Geometry: final body of the model. Coordinates: model frame, mm. Face numbers are marked on the shaded views. A direction names the side the tool comes from. Round coordinates to 2 decimals unless told otherwise and drop trailing zeros. Write each loop counter-clockwise with the first axis right and the second up, starting at its lowest first coordinate (ties: lowest second). Pieces come first, ordered by that corner, then holes. Notation, with made-up numbers: M 40,-18 L 92,-18 A16 cw 92,0 Z; hole C 68.25,-13 d11. An arc over 180 degrees is marked long. Answer as CSV lines item,"result". Start each with the question number.
Q1. Ray query, probe 1 along Z at (x, y) = (2.35, -0.3); probe 2 along Z at (x, y) = (-1.85, 1.6); probe 3 along X at (y, z) = (-0.9, 1.75). Return the intervals inside material, ascending.
Q2. Reachability of the marked faces 4, 5 and 6 from +Z, -Z, +X, -X, +Y, -Y: full face, straight path, thin tool, end or side. Return the list, or none.
Q3. Section query C-C on z = 3.5. Output: boundary loops of the cut face in (x, y).
Q4. Section query B-B on x = 1.15. Output: boundary loops of the cut face in (y, z).
Q5. Section query D-D on z = 0. Output: boundary loops of the cut face in (x, y).
Q6. First-contact query: pin 1 (2.5 mm diameter, centred on x = 0, y = 0, fed in from -Z); pin 2 (2 mm diameter, centred on y = 0.5, z = -2.5, fed in from -X); pin 3 (2 mm diameter, centred on y = -1.5, z = 2.5, fed in from +X). Flat tips, straight axial feed; report the tip coordinate or a pass-through.
Q7. Mould query, pull axis Z, two halves, no side actions, for the marked faces 1, 2 and 3. Classes: pulls with the +Z half, pulls with the -Z half, needs draft (parallel to the pull), parting line crosses it, or undercut.
Q8. Section query A-A on y = 0. Output: boundary loops of the cut face in (x, z), and give its area (3 significant figures).
```python
from build123d import *


with BuildPart() as part:
    # Sketch1 → Revolve1 (revolve)
    with BuildSketch(Plane(origin=(0, 0, 0), x_dir=(1, 0, 0), z_dir=(0, 1, 0))):
        with BuildLine():
            Line((1.4732, 4.0005), (1.4732, -4.0005))
            Line((1.4732, -4.0005), (2.4892, -4.0005))
            Line((2.4892, -4.0005), (2.4892, -3.1115))
            Line((2.4892, -3.1115), (1.9304, -3.1115))
            Line((1.9304, -3.1115), (1.9304, -2.0955))
            ThreePointArc((1.9304, -2.0955), (2.849133975, 0), (1.9304, 2.0955))
            Line((1.9304, 2.0955), (1.9304, 3.1115))
            Line((1.9304, 3.1115), (2.4892, 3.1115))
            Line((2.4892, 3.1115), (2.4892, 4.0005))
            Line((2.4892, 4.0005), (1.4732, 4.0005))
        make_face()
    revolve(axis=Axis((0, 0, -2.773013621), (0, 0, 1)))


solid = part.part
```
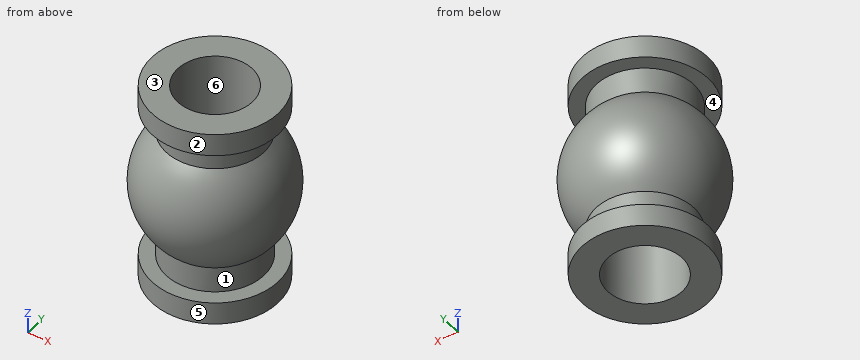
Entries:
1,probe 1,"z = -4 to -3.11, -1.58 to 1.58, 3.11 to 4"
1,probe 2,"z = -4 to -3.11, -1.46 to 1.46, 3.11 to 4"
1,probe 3,"x = -2.06 to -1.17, 1.17 to 2.06"
2,face 4,"none"
2,face 5,"-Z"
2,face 6,"+Z, -Z"
3,outline,"C 0,0 d4.98; hole C 0,0 d2.95"
4,outline,"M -2.21,-4 L -0.92,-4 L -0.92,4 L -2.21,4 L -2.21,3.11 L -1.55,3.11 L -1.55,2.1 A2.61 ccw -1.55,-2.1 L -1.55,-3.11 L -2.21,-3.11 Z; M 0.92,-4 L 2.21,-4 L 2.21,-3.11 L 1.55,-3.11 L 1.55,-2.1 A2.61 ccw 1.55,2.1 L 1.55,3.11 L 2.21,3.11 L 2.21,4 L 0.92,4 Z"
5,outline,"C 0,0 d5.7; hole C 0,0 d2.95"
6,pin 1,"passes through"
6,pin 2,"stops at x = -2.49"
6,pin 3,"stops at x = 2.39"
7,face 1,"undercut"
7,face 2,"needs draft"
7,face 3,"pulls with the +Z half"
8,outline,"M -2.49,-4 L -1.47,-4 L -1.47,4 L -2.49,4 L -2.49,3.11 L -1.93,3.11 L -1.93,2.1 A2.85 ccw -1.93,-2.1 L -1.93,-3.11 L -2.49,-3.11 Z; M 1.47,-4 L 2.49,-4 L 2.49,-3.11 L 1.93,-3.11 L 1.93,-2.1 A2.85 ccw 1.93,2.1 L 1.93,3.11 L 2.49,3.11 L 2.49,4 L 1.47,4 Z"
8,area,"14.6 mm^2"
